```python
from build123d import *

# Parameters (mm, degrees)
SKETCH2_W                = 38.1
SKETCH2_H                = 24.13
BOSS_EXTRUDE1_DEPTH      = 5.08
SKETCH3_W                = 23.876
SKETCH3_H                = 13.208
CUT_EXTRUDE1_DEPTH       = 5.08
BOSS_EXTRUDE2_DEPTH      = 34.154802
BOSS_EXTRUDE2_DEPTH_BACK = 78.16772
SKETCH4_W                = 5.08
SKETCH4_H                = 10.16
CUT_EXTRUDE2_REACH       = 87.366
SKETCH5_R                = 1.27


with BuildPart() as part:
    # Sketch2 → Boss-Extrude1 (new body)
    with BuildSketch(Plane.XY):
        Rectangle(SKETCH2_W, SKETCH2_H)
    extrude(amount=BOSS_EXTRUDE1_DEPTH)

    # Sketch3 → Cut-Extrude1 (cut)
    with BuildSketch(Plane.XY.offset(5.08)):
        Rectangle(SKETCH3_W, SKETCH3_H)
    extrude(amount=-CUT_EXTRUDE1_DEPTH, mode=Mode.SUBTRACT)

    # Sketch4 → Boss-Extrude2 (add, two sides: drawn at the far end of the back side and taken through both)
    with BuildSketch(Plane.XY.offset(5.08).offset(-BOSS_EXTRUDE2_DEPTH_BACK)):
        with Locations((-16.51, -17.145)):
            Rectangle(SKETCH4_W, SKETCH4_H)
    extrude(amount=BOSS_EXTRUDE2_DEPTH + BOSS_EXTRUDE2_DEPTH_BACK)

    # Sketch5 → Cut-Extrude2 (cut, up to next)
    with BuildSketch(Plane.ZY.offset(19.05), mode=Mode.PRIVATE) as cut_extrude2_sk1:
        with Locations((-68.007719547, -17.145)):
            Circle(SKETCH5_R)
    cut_extrude2_tool1 = extrude(cut_extrude2_sk1.sketch, amount=-CUT_EXTRUDE2_REACH, mode=Mode.PRIVATE) & part.part
    # Sketch5 → Cut-Extrude2 (cut, up to next)
    with BuildSketch(Plane.ZY.offset(19.05), mode=Mode.PRIVATE) as cut_extrude2_sk2:
        with Locations((34.154802315, -17.145)):
            Circle(SKETCH5_R)
    cut_extrude2_tool2 = extrude(cut_extrude2_sk2.sketch, amount=-CUT_EXTRUDE2_REACH, mode=Mode.PRIVATE) & part.part
    add(cut_extrude2_tool1.solids().sort_by_distance((-19.05, -17.145, -68.00772))[0], mode=Mode.SUBTRACT)
    add(cut_extrude2_tool2.solids().sort_by_distance((-19.05, -17.145, 34.154802))[0], mode=Mode.SUBTRACT)


solid = part.part
```
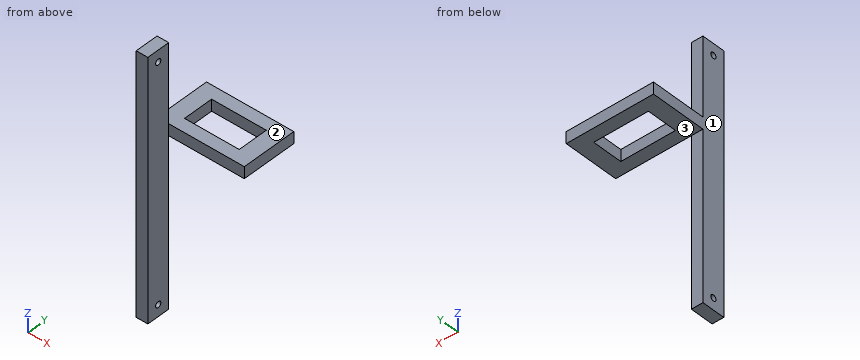
Design review of the part built by this model. Coordinates are the model's own, in mm. Face numbers are marked on the shaded views. Give positions to 0.01 mm unless a question says otherwise; leave off trailing zeros. Write each loop counter-clockwise with the first axis right and the second up, starting at its lowest first coordinate (ties: lowest second). Pieces come first, ordered by that corner, then holes. Notation, with made-up numbers: (41.5, 70.5) -> (56.5, 70.5) arc R28 cw to (56.5, 98.5) -> close; hole circle Ø10 at (64, -17.5). An arc over 180 degrees is marked (long way). Answer in a Markdown table with one row per item.
(1) Consider section A-A (y = 1.5). State the section outline as (x, z) points.
Results:
| item | result |
|---|---|
| outline | (-19.05, 0) -> (-11.94, 0) -> (-11.94, 5.08) -> (-19.05, 5.08) -> close; (11.94, 0) -> (19.05, 0) -> (19.05, 5.08) -> (11.94, 5.08) -> close |
(2) Mouldability with a two-part tool opening along Z and no side actions: class the marked faces 1, 2 and 3 as +Z half, -Z half, draft (parallel to the pull), parting line (faces both ways), or undercut.
Results:
| item | result |
|---|---|
| face 1 | draft |
| face 2 | +Z half |
| face 3 | -Z half |
(3) Consider section D-D (x = -15.5). State the section outline as (y, z) points (3 decimals).
Results:
| item | result |
|---|---|
| outline | (-22.225, -73.088) -> (-12.065, -73.088) -> (-12.065, 0) -> (12.065, 0) -> (12.065, 5.08) -> (-12.065, 5.08) -> (-12.065, 39.235) -> (-22.225, 39.235) -> close; hole circle Ø2.54 at (-17.145, -68.008); hole circle Ø2.54 at (-17.145, 34.155) |
(4) Consider section C-C (z = 4). State the section outline as (x, y) points (3 decimals).
Results:
| item | result |
|---|---|
| outline | (-19.05, -22.225) -> (-13.97, -22.225) -> (-13.97, -12.065) -> (19.05, -12.065) -> (19.05, 12.065) -> (-19.05, 12.065) -> close; hole (-11.938, -6.604) -> (11.938, -6.604) -> (11.938, 6.604) -> (-11.938, 6.604) -> close |
(5) To check wall thickness, follow probe 1 along Y at (x, z) = (-11.5, 5) (3 decimals); probe 2 along Y at (x, z) = (-16.5, -28.5) (3 decimals); probe 3 along Z at (x, y) = (-12, -3.5). State the ranges of each line that lie inside material, in increasing order.
Results:
| item | result |
|---|---|
| probe 1 | -12.065 to -6.604, 6.604 to 12.065 |
| probe 2 | -22.225 to -12.065 |
| probe 3 | 0 to 5.08 |
(6) Consider section B-B (x = -8). State the section outline as (y, z) points (3 decimals).
Results:
| item | result |
|---|---|
| outline | (-12.065, 0) -> (-6.604, 0) -> (-6.604, 5.08) -> (-12.065, 5.08) -> close; (6.604, 0) -> (12.065, 0) -> (12.065, 5.08) -> (6.604, 5.08) -> close |
(7) Clearance check with flat-ended pins moving along their axes: pin 1 (6 mm diameter, centred on y = -5, z = 7, fed in from -X); pin 2 (12 mm diameter, centred on x = -8, y = -3.5, fed in from -Z); pin 3 (8 mm diameter, centred on x = 14.5, y = -2, fed in from +Z); pin 4 (2.5 mm diameter, centred on x = 5, z = 3, fed in from -Y) (3 decimals). State where each tip first meets the part, or that it passes through.
Results:
| item | result |
|---|---|
| pin 1 | x = -19.05 |
| pin 2 | z = 0 |
| pin 3 | z = 5.08 |
| pin 4 | y = -12.065 |
